Here's how the part is built. I have some questions about the finished solid (model axes, mm). A direction names the side the tool comes from. Round coordinates to 2 decimals unless told otherwise and drop trailing zeros. Write each loop counter-clockwise with the first axis right and the second up, starting at its lowest first coordinate (ties: lowest second). Pieces come first, ordered by that corner, then holes. Notation, with made-up numbers: (-3.75, 15.25) - (32.25, 15.25) arc R24 ccw to (32.25, 43.25) - close; hole circle Ø3 at (-15, 43). An arc over 180 degrees is marked (long way). One line per item, written item: value. Start each with the question number.
Item 1: Imagine slicing it at D-D, the plane z = -41. Please give me the cut outline in (x, y), then the cut area to 3 significant figures.
Item 2: For P1, Ø0.8, axis at y = -12, z = -49.5, coming from the -X side; P2, Ø7.5, axis at x = 3, y = 6, coming from the -Z side; P3, Ø0.8, axis at y = 63, z = -49, coming from the +X side, each with a flat end and sliding along its axis, tell me the tip position at first contact or that it passes through.
Item 3: If I drill on line 1 (Y direction, x = 8, z = 0.6); line 2 (X direction, y = 1, z = -66.5); line 3 (Y direction, x = 0, z = -65), over which ranges is the centre line in solid material (lowest first)?
Item 4: Imagine slicing it at A-A, the plane z = -13. Please give me the cut outline in (x, y), then the cut area to 3 significant figures.
Item 5: Thinking about a two-plate mould opening in Z: for faces 4 (the face through (5.5, 6, -3)), 5 (the face through (-10.7, 26, -68)), 6 (the face through (19, 44, -1)), which applies, released by +Z, released by -Z, zero draft, split by the parting line, or undercut?
Item 6: For faces 1 (the face through (58.33, 26.1, -106.95)), 2 (the face through (49.169, 6.876, -2.198)), 3 (the face through (24.62, 49.68, -0.87)), which set-ups out of +Z, -Z, +X, -X, +Y, -Y let a thin tool reach every point of the face, with its end or its side?
Item 7: Imagine slicing it at B-B, the plane y = 26. Please give me the cut outline in (x, z), then the cut area to 3 significant figures.
Item 8: Imagine slicing it at C-C, the plane x = 25.3. Count the separate pieces of the cut face and the enclosed holes in it, then the cut area to 3 significant figures.
```python
from build123d import *

# Parameters (mm, degrees)
SKETCH1_R           = 5
SKETCH1_W           = 39
SKETCH1_H           = 20
BOSS_EXTRUDE1_DEPTH = 1.5
BOSS_EXTRUDE3_START = 133.5
BOSS_EXTRUDE3_DEPTH = 133.5
BOSS_EXTRUDE4_DEPTH = 30
CUT_EXTRUDE1_DEPTH  = 15
CUT_EXTRUDE2_DEPTH  = 15
SKETCH7_R           = 2
CUT_EXTRUDE3_DEPTH  = 15
SKETCH10_W          = 45
SKETCH10_H          = 70
CUT_EXTRUDE4_DEPTH  = 1.5
SKETCH11_R          = 2
CUT_EXTRUDE6_DEPTH  = 1.5
SKETCH15_W          = 7
SKETCH15_H          = 7
SKETCH15_W_2        = 5.9
SKETCH15_H_2        = 8
BOSS_EXTRUDE5_DEPTH = 6
SKETCH16_R          = 2.25
SKETCH16_R_2        = 1.75
CUT_EXTRUDE20_DEPTH = 10
FILLET5_R           = 5
FILLET6_R           = 5
FILLET7_R           = 5
SKETCH17_W          = 4.5
SKETCH17_H          = 1.5
BOSS_EXTRUDE6_DEPTH = 135


with BuildPart() as part:
    # Sketch1 → Boss-Extrude1 (new body)
    with BuildSketch(Plane.XY):
        with BuildLine():
            Line((50.3, -11.5), (0.3, -11.5))
            ThreePointArc((0.3, -11.5), (-8.538834765, -7.838834765), (-12.2, 1))
            Line((-12.2, 1), (-12.2, 51))
            ThreePointArc((-12.2, 51), (-8.538834765, 59.838834765), (0.3, 63.5))
            Line((0.3, 63.5), (50.3, 63.5))
            ThreePointArc((50.3, 63.5), (59.138834765, 59.838834765), (62.8, 51))
            Line((62.8, 51), (62.8, 1))
            ThreePointArc((62.8, 1), (59.138834765, -7.838834765), (50.3, -11.5))
        make_face()
        with Locations((8, 34)):
            Circle(SKETCH1_R, mode=Mode.SUBTRACT)
        with Locations((25.3, 12.5)):
            Rectangle(SKETCH1_W, SKETCH1_H, mode=Mode.SUBTRACT)
    extrude(amount=BOSS_EXTRUDE1_DEPTH)

    # Sketch3 → Boss-Extrude3 (add)
    with BuildSketch(Plane(origin=(0, 0, 0), x_dir=(-1, 0, 0), z_dir=(0, 0, -1)).offset(BOSS_EXTRUDE3_START)):
        with BuildLine():
            Line((-50.3, 63.5), (-0.3, 63.5))
            ThreePointArc((-0.3, 63.5), (8.538834765, 59.838834765), (12.2, 51))
            Line((12.2, 51), (12.2, 1))
            ThreePointArc((12.2, 1), (8.538834765, -7.838834765), (-0.3, -11.5))
            Line((-0.3, -11.5), (-50.3, -11.5))
            ThreePointArc((-50.3, -11.5), (-59.138834765, -7.838834765), (-62.8, 1))
            Line((-62.8, 1), (-62.8, 51))
            ThreePointArc((-62.8, 51), (-59.138834765, 59.838834765), (-50.3, 63.5))
        make_face()
        with BuildLine():
            Line((10.7, 1), (10.7, 51))
            ThreePointArc((10.7, 51), (7.478174593, 58.778174593), (-0.3, 62))
            Line((-0.3, 62), (-50.3, 62))
            ThreePointArc((-50.3, 62), (-58.078174593, 58.778174593), (-61.3, 51))
            Line((-61.3, 51), (-61.3, 1))
            ThreePointArc((-61.3, 1), (-58.078174593, -6.778174593), (-50.3, -10))
            Line((-50.3, -10), (-0.3, -10))
            ThreePointArc((-0.3, -10), (7.478174593, -6.778174593), (10.7, 1))
        make_face(mode=Mode.SUBTRACT)
    extrude(amount=-BOSS_EXTRUDE3_DEPTH)

    # Sketch4 → Boss-Extrude4 (add)
    with BuildSketch(Plane(origin=(0, 0, -132), x_dir=(-1, 0, 0), z_dir=(0, 0, -1))):
        with BuildLine():
            Line((-61.3, 33), (-61.3, 19))
            add(Edge.make_bspline(
                [(-57.8, 22), (-60.735988769, 21.788932059), (-61.3, 19)],
                knots=[0, 0, 0, 1, 1, 1], degree=2))
            ThreePointArc((-57.8, 22), (-53.8, 26), (-57.8, 30))
            add(Edge.make_bspline(
                [(-57.8, 30), (-60.735988769, 30.211067941), (-61.3, 33)],
                knots=[0, 0, 0, 1, 1, 1], degree=2))
        make_face()
        with BuildLine():
            Line((10.7, 33), (10.7, 19))
            add(Edge.make_bspline(
                [(7.2, 22), (10.135988769, 21.788932059), (10.7, 19)],
                knots=[0, 0, 0, 1, 1, 1], degree=2))
            ThreePointArc((7.2, 22), (3.2, 26), (7.2, 30))
            add(Edge.make_bspline(
                [(7.2, 30), (10.135988769, 30.211067941), (10.7, 33)],
                knots=[0, 0, 0, 1, 1, 1], degree=2))
        make_face()
    extrude(amount=-BOSS_EXTRUDE4_DEPTH)

    # Sketch5 → Cut-Extrude1 (cut)
    with BuildSketch(Plane(origin=(0, 33, 0), x_dir=(-1, 0, 0), z_dir=(0, -1, 0))):
        Polygon((10.7, 102), (3.2, 102), (3.2, 114.5), align=None)
    extrude(amount=CUT_EXTRUDE1_DEPTH, mode=Mode.SUBTRACT)

    # Sketch6 → Cut-Extrude2 (cut)
    with BuildSketch(Plane(origin=(0, 33, 0), x_dir=(-1, 0, 0), z_dir=(0, -1, 0))):
        Polygon((-61.3, 102), (-53.8, 102), (-53.8, 114.5), align=None)
    extrude(amount=CUT_EXTRUDE2_DEPTH, mode=Mode.SUBTRACT)

    # Sketch7 → Cut-Extrude3 (cut)
    with BuildSketch(Plane(origin=(0, 0, -132), x_dir=(-1, 0, 0), z_dir=(0, 0, -1))):
        with Locations((-57.8, 26)):
            Circle(SKETCH7_R)
        with Locations((7.2, 26)):
            Circle(SKETCH7_R)
    extrude(amount=-CUT_EXTRUDE3_DEPTH, mode=Mode.SUBTRACT)

    # Sketch10 → Cut-Extrude4 (cut)
    with BuildSketch(Plane(origin=(0, 63.5, 0), x_dir=(1, 0, 0), z_dir=(0, 1, 0))):
        with Locations((25.3, 63.5)):
            Rectangle(SKETCH10_W, SKETCH10_H)
    extrude(amount=-CUT_EXTRUDE4_DEPTH, mode=Mode.SUBTRACT)

    # Sketch11 → Cut-Extrude6 (cut)
    with BuildSketch(Plane(origin=(0, 63.5, 0), x_dir=(1, 0, 0), z_dir=(0, 1, 0))):
        with Locations(Location((25.3, 102.5, 0), (0, 0, 270))):
            Circle(SKETCH11_R)
        with Locations(Location((25.3, 24.5, 0), (0, 0, 270))):
            Circle(SKETCH11_R)
    extrude(amount=-CUT_EXTRUDE6_DEPTH, mode=Mode.SUBTRACT)

    # Sketch15 → Boss-Extrude5 (add)
    with BuildSketch(Plane.XY):
        with Locations((24.5, 44)):
            Rectangle(SKETCH15_W, SKETCH15_H)
        with Locations((48.55, 6.35)):
            Rectangle(SKETCH15_W_2, SKETCH15_H_2)
        with Locations((2, 6.35)):
            Rectangle(SKETCH15_W, SKETCH15_H_2)
    extrude(amount=-BOSS_EXTRUDE5_DEPTH)

    # Sketch16 → Cut-Extrude20 (cut)
    with BuildSketch(Plane.XY.offset(1.5)):
        with Locations((25, 43.5)):
            Circle(SKETCH16_R)
        with Locations((47.5, 6.35)):
            Circle(SKETCH16_R_2)
        with Locations((2.5, 6.35)):
            Circle(SKETCH16_R)
    extrude(amount=-CUT_EXTRUDE20_DEPTH, mode=Mode.SUBTRACT)

    # Fillet5
    fillet5_edges = [part.edges().sort_by_distance(p)[0] for p in [
        (-1.5, 6.35, 0),
        (2, 2.35, 0),
        (2, 10.35, 0),
    ]]
    fillet(fillet5_edges, radius=FILLET5_R)

    # Fillet6
    fillet6_edges = [part.edges().sort_by_distance(p)[0] for p in [
        (51.5, 6.35, 0),
        (48.55, 10.35, 0),
        (48.55, 2.35, 0),
    ]]
    fillet(fillet6_edges, radius=FILLET6_R)

    # Fillet7
    fillet7_edges = [part.edges().sort_by_distance(p)[0] for p in [
        (21, 44, 0),
        (24.5, 40.5, 0),
        (28, 44, 0),
        (24.5, 47.5, 0),
    ]]
    fillet(fillet7_edges, radius=FILLET7_R)

    # Sketch17 → Boss-Extrude6 (add)
    with BuildSketch(Plane.XY.offset(1.5)):
        with Locations((41.55, -12.25)):
            Rectangle(SKETCH17_W, SKETCH17_H)
        with Locations((9.05, -12.25)):
            Rectangle(SKETCH17_W, SKETCH17_H)
    extrude(amount=-BOSS_EXTRUDE6_DEPTH)


solid = part.part
```
Values follow:
1. outline: (-12.2, 1) arc R12.5 ccw to (0.3, -11.5) - (6.8, -11.5) - (6.8, -13) - (11.3, -13) - (11.3, -11.5) - (39.3, -11.5) - (39.3, -13) - (43.8, -13) - (43.8, -11.5) - (50.3, -11.5) arc R12.5 ccw to (62.8, 1) - (62.8, 51) arc R12.5 ccw to (50.3, 63.5) - (47.8, 63.5) - (47.8, 62) - (50.3, 62) arc R11 cw to (61.3, 51) - (61.3, 1) arc R11 cw to (50.3, -10) - (0.3, -10) arc R11 cw to (-10.7, 1) - (-10.7, 51) arc R11 cw to (0.3, 62) - (2.8, 62) - (2.8, 63.5) - (0.3, 63.5) arc R12.5 ccw to (-12.2, 51) - close
1. area: 357 mm^2
2. P1: stops at x = 6.8
2. P2: stops at z = -6
2. P3: stops at x = 54.96
3. line 1: y = -13 to 2.5, 22.5 to 29, 39 to 63.5
3. line 2: x = -12.2 to -10.7, 61.3 to 62.8
3. line 3: y = -11.5 to -10, 62 to 63.5
4. outline: (-12.2, 1) arc R12.5 ccw to (0.3, -11.5) - (6.8, -11.5) - (6.8, -13) - (11.3, -13) - (11.3, -11.5) - (39.3, -11.5) - (39.3, -13) - (43.8, -13) - (43.8, -11.5) - (50.3, -11.5) arc R12.5 ccw to (62.8, 1) - (62.8, 51) arc R12.5 ccw to (50.3, 63.5) - (0.3, 63.5) arc R12.5 ccw to (-12.2, 51) - close; hole (-10.7, 1) arc R11 ccw to (0.3, -10) - (50.3, -10) arc R11 ccw to (61.3, 1) - (61.3, 51) arc R11 ccw to (50.3, 62) - (0.3, 62) arc R11 ccw to (-10.7, 51) - close
4. area: 424 mm^2
5. face 4: zero draft
5. face 5: undercut
5. face 6: released by -Z
6. face 1: none
6. face 2: +Z, -Z
6. face 3: -Z
7. outline: (-12.2, -133.5) - (-10.7, -133.5) - (-10.7, -132) - (-9.2, -132) - (-9.2, -117) - (-5.2, -117) - (-5.2, -132) - (-3.2, -132) - (-3.2, -114.5) - (-10.7, -102) - (-10.7, 0) - (61.3, 0) - (61.3, -102) - (53.8, -114.5) - (53.8, -132) - (55.8, -132) - (55.8, -117) - (59.8, -117) - (59.8, -132) - (61.3, -132) - (61.3, -133.5) - (62.8, -133.5) - (62.8, 1.5) - (-12.2, 1.5) - close
7. area: 749 mm^2
8. separate pieces: 6
8. enclosed holes: 0
8. area: 385 mm^2
